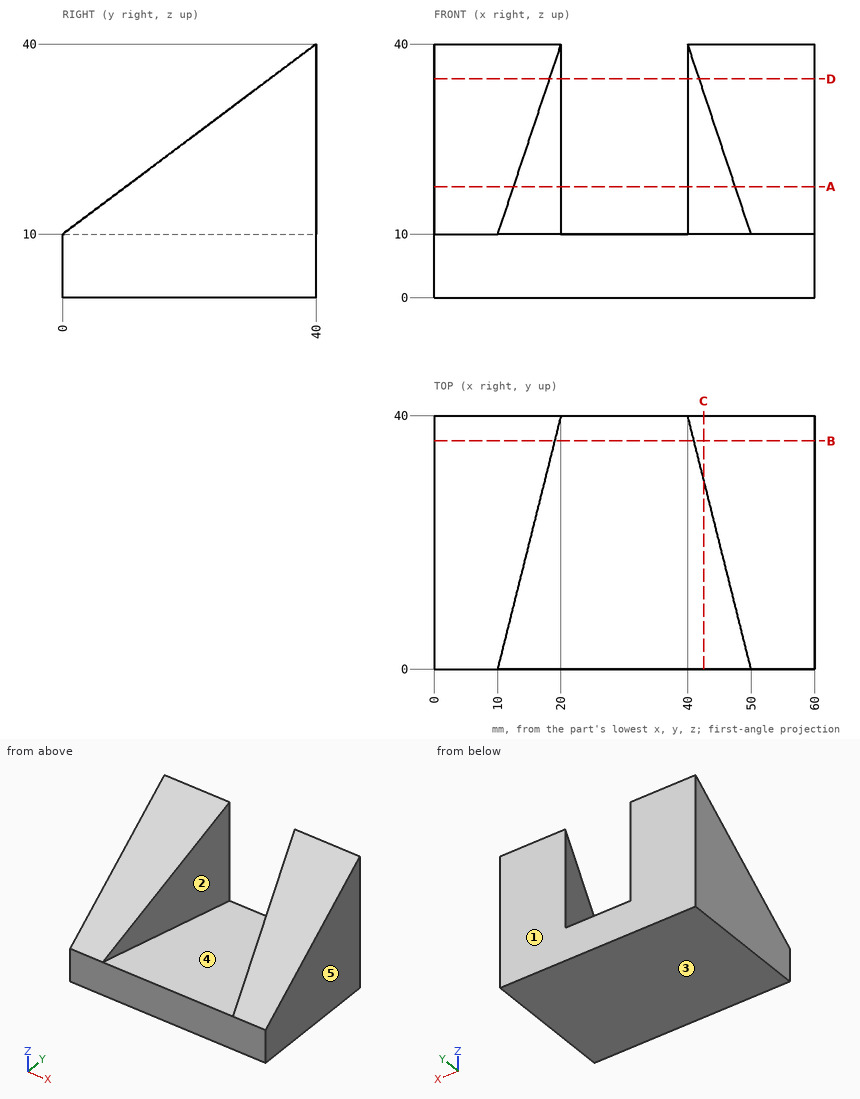
Check sheet for the drawn part. Datum: minimum x, y, z corner. Units: mm. A direction names the side the tool comes from. Coordinates: 2 decimals unless noted, no trailing zeros. Loops run counter-clockwise (first coordinate to the right, second up) from the corner with the lowest first, then second, coordinate; pieces in that order, holes last. Notation, with made-up numbers: (42.5, 30) -> (76.5, 30) arc R24 ccw to (76.5, 46) -> close; hole circle Ø6 at (89.5, 74.5). An arc over 180 degrees is marked (long way). Answer in a Markdown table with one row per item.
1. Go/stop test with flat-tipped pins: pin 1 (3 mm diameter, centred on x = 9, y = 19.5, fed in from -Z); pin 2 (6 mm diameter, centred on x = 7, z = 34, fed in from -Y). Record where each tip stops, or that it passes through.
Check values:
| item | result |
|---|---|
| pin 1 | stops at z = 0 |
| pin 2 | stops at y = 28 |
2. Sectioned sample at B-B, the plane y = 36. Record the boundary of the cut face in (x, z).
Check values:
| item | result |
|---|---|
| outline | (0, 0) -> (60, 0) -> (60, 37) -> (41, 37) -> (41, 10) -> (19, 10) -> (19, 37) -> (0, 37) -> close |
3. Sectioned sample at C-C, the plane x = 42.5. Record the boundary of the cut face in (y, z), then the cut area to 4 significant figures.
Check values:
| item | result |
|---|---|
| outline | (0, 0) -> (40, 0) -> (40, 40) -> (30, 32.5) -> (30, 10) -> (0, 10) -> close |
| area | 662.5 mm2 |
4. Release check for a two-part mould opening along X. For the marked faces 3, 4 and 5 record: released by +X, released by -X, zero draft, split by the parting line, or undercut.
Check values:
| item | result |
|---|---|
| face 3 | zero draft |
| face 4 | undercut |
| face 5 | released by +X |
5. Sectioned sample at A-A, the plane z = 17.5. Record the boundary of the cut face in (x, y), then the cut area to 3 significant figures.
Check values:
| item | result |
|---|---|
| outline | (0, 10) -> (12.5, 10) -> (20, 40) -> (0, 40) -> close; (40, 40) -> (47.5, 10) -> (60, 10) -> (60, 40) -> close |
| area | 975 mm2 |
6. Access from +Z, -Z, +X, -X, +Y, -Y to the whole of each face (thin tool, end or side, straight path). Record for the marked faces 1 and 2.
Check values:
| item | result |
|---|---|
| face 1 | +Z, -Z, +X, -X, +Y |
| face 2 | +Z, -Y |
7. Sectioned sample at D-D, the plane z = 34.5. Record the boundary of the cut face in (x, y).
Check values:
| item | result |
|---|---|
| outline | (0, 32.67) -> (18.17, 32.67) -> (20, 40) -> (0, 40) -> close; (40, 40) -> (41.83, 32.67) -> (60, 32.67) -> (60, 40) -> close |
8. Material ranges on line 1 along Z through (x, y) = (29, 34); line 2 along X through (y, z) = (38.5, 22) (3 decimals); line 3 along X through (y, z) = (23, 21.5), recorded low to high. Write a range as [from, to].
Check values:
| item | result |
|---|---|
| line 1 | z = [0, 10] |
| line 2 | x = [0, 19.625], [40.375, 60] |
| line 3 | x = [0, 15.75], [44.25, 60] |
